Could you check a few things on this model? Use its own coordinates, in mm. Face numbers are marked on the shaded views. A direction names the side the tool comes from. Give positions to 0.01 mm unless a question says otherwise; leave off trailing zeros. Loops run counter-clockwise (first coordinate to the right, second up) from the corner with the lowest first, then second, coordinate; pieces in that order, holes last. Notation, with made-up numbers: M 55,-34 L 65,-34 A29 ccw 65,-9 Z; hole C 2,63.25 d6. An arc over 180 degrees is marked long. Return JSON: item names as keys, results as strings. Group by question number.
1. If we section it at B-B (x = 0): Write out the boundary of the cut face in (y, z).
2. For the marked faces 5 and 6, which set-ups out of +Z, -Z, +X, -X, +Y, -Y let a thin tool reach every point of the face, with its end or its side?
3. If we mould it in two halves opening along Y, with no side actions, what happens to the marked faces 1, 2, 3 and 4? For each: +Y half, -Y half, draft (parallel to the pull), parting line (faces both ways), or undercut.
4. If we section it at D-D (x = 8): Write out the boundary of the cut face in (y, z).
5. For pin 1 (1.2 mm diameter, centred on x = 0, y = 4.5, fed in from -Z); pin 2 (1.5 mm diameter, centred on x = 2.5, z = -2, fed in from -Y); pin 3 (4 mm diameter, centred on y = 7.5, z = -4, fed in from -X), each with a flat end and sliding along its axis, tell me the tip position at first contact or that it passes through.
6. Please list where these lines run through material, in increasing order: line 1 (Y direction, x = 0, z = -2.1); line 2 (Y direction, x = -1.5, z = -3); line 3 (X direction, y = -0.25, z = -5.25).
7. If we section it at C-C (z = -1.25): Write out the boundary of the cut face in (x, y), plus the area to 3 significant figures.
8. If we section it at A-A (y = 0): Write out the boundary of the cut face in (x, z).
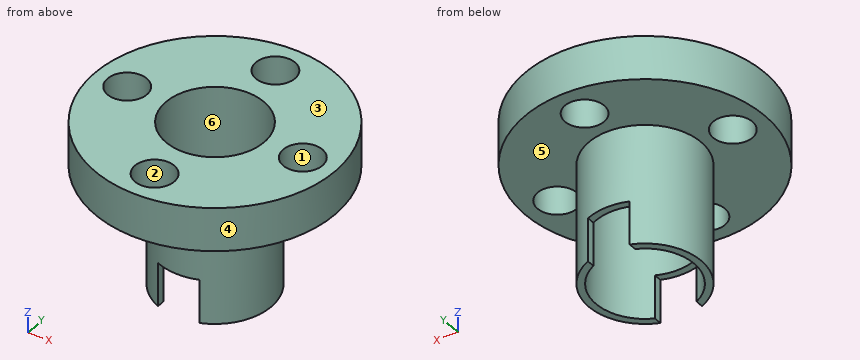
```python
from build123d import *

# Parameters (mm, degrees)
SKETCH001_R   = 4.5
HOLE_DEPTH    = 25
SKETCH002_W   = 3.8
SKETCH002_H   = 4
POCKET_DEPTH  = 10
SKETCH003_R   = 1.8
HOLE001_DEPTH = 25


with BuildPart() as part:
    # Sketch → Revolution (revolve)
    with BuildSketch(Plane.XZ):
        Polygon((0, 0), (11, 0), (11, -4), (5.15, -4), (5.15, -15), (0, -15), align=None)
    revolve(axis=Axis((0, 0, 0), (0, 0, 1)))

    # Sketch001 (on Face1 of Revolution) → Hole (cut)
    with BuildSketch(Plane(origin=(0, 0, 0), x_dir=(-1, 0, 0), z_dir=(0, 0, 1))):
        Circle(SKETCH001_R)
    extrude(amount=-HOLE_DEPTH, mode=Mode.SUBTRACT)

    # Sketch002 → Pocket (cut, symmetric)
    with BuildSketch(Plane.XZ):
        with Locations((0, -13)):
            Rectangle(SKETCH002_W, SKETCH002_H)
    extrude(amount=POCKET_DEPTH, both=True, mode=Mode.SUBTRACT)

    # Sketch003 (on Face1 of Pocket) → Hole001 (cut)
    with BuildSketch(Plane(origin=(0, 0, 0), x_dir=(-1, 0, 0), z_dir=(0, 0, 1))):
        with Locations((0, 8)):
            Circle(SKETCH003_R)
        with Locations((-8, 0)):
            Circle(SKETCH003_R)
        with Locations((0, -8)):
            Circle(SKETCH003_R)
        with Locations((8, 0)):
            Circle(SKETCH003_R)
    extrude(amount=-HOLE001_DEPTH, mode=Mode.SUBTRACT)


solid = part.part
```
Answer:
{
 "1": {"outline": "M -11,-4 L -9.8,-4 L -9.8,0 L -11,0 Z; M -6.2,-4 L -5.15,-4 L -5.15,-11 L -4.5,-11 L -4.5,0 L -6.2,0 Z; M 4.5,-11 L 5.15,-11 L 5.15,-4 L 6.2,-4 L 6.2,0 L 4.5,0 Z; M 9.8,-4 L 11,-4 L 11,0 L 9.8,0 Z"},
 "2": {"face 5": "-Z", "face 6": "+Z, -Z"},
 "3": {"face 1": "undercut", "face 2": "undercut", "face 3": "draft", "face 4": "parting line"},
 "4": {"outline": "M -7.55,-4 L -1.8,-4 L -1.8,0 L -7.55,0 Z; M 1.8,-4 L 7.55,-4 L 7.55,0 L 1.8,0 Z"},
 "5": {"pin 1": "stops at z = -11", "pin 2": "stops at y = -10.86", "pin 3": "stops at x = -9.53"},
 "6": {"line 1": "y = -11 to -9.8, -6.2 to -4.5, 4.5 to 6.2, 9.8 to 11", "line 2": "y = -10.9 to -8.99, -7.01 to -4.24, 4.24 to 7.01, 8.99 to 10.9", "line 3": "x = -5.14 to -4.49, 4.49 to 5.14"},
 "7": {"outline": "C 0,0 d22; hole C -8,0 d3.6; hole C 0,0 d9; hole C 0,-8 d3.6; hole C 0,8 d3.6; hole C 8,0 d3.6", "area": "276 mm²"},
 "8": {"outline": "M -11,-4 L -9.8,-4 L -9.8,0 L -11,0 Z; M -6.2,-4 L -5.15,-4 L -5.15,-15 L -4.5,-15 L -4.5,0 L -6.2,0 Z; M 4.5,-15 L 5.15,-15 L 5.15,-4 L 6.2,-4 L 6.2,0 L 4.5,0 Z; M 9.8,-4 L 11,-4 L 11,0 L 9.8,0 Z"}
}
